Verification items for the finished model (mm, model axes). A direction names the side the tool comes from. Round coordinates to 2 decimals unless told otherwise and drop trailing zeros. Order: outer loops, then holes, each group sorted by start corner. A loop starts at its lowest first (then second) coordinate and runs counter-clockwise, first axis right, second up. Notation, with made-up numbers: M 74,13.25 L 117,13.25 A16 cw 117,43.25 Z; hole C 43,0 d1. An arc over 180 degrees is marked long. Use one line per item in the form item = value. Start each with the question number.
Item 1: Go/stop test with flat-tipped pins: pin 1 Ø0.5 at (y, z) = (4.5, 7.5) entering from +X; pin 2 Ø0.7 at (x, z) = (-4.5, 5) entering from +Y; pin 3 Ø2.5 at (x, z) = (0, 5) entering from +Y. Record where each tip stops, or that it passes through.
Item 2: Release check for a two-part mould opening along X. For faces 4 (the cylindrical face through (0.46, 2.47, 7.05)), 5 (the cylindrical face through (3.97, 1.97, 9.94)), 6 (the flat face through (1.3, 5, 2.8)) record: +X half, -X half, draft (parallel to the pull), parting line (faces both ways), or undercut.
Item 3: Thickness scan on probe 1 along Z at (x, y) = (0, 3.15); probe 2 along X at (y, z) = (2.05, 5); probe 3 along X at (y, z) = (3.75, 5). Record the ranges inside material, lowest first. Write a range as [from, to].
Item 4: Cross-section at B-B on z = 5. Enter the section's corners in (x, y), then the cut area to 3 significant figures.
Item 5: Tool access check on faces 1 (the flat face through (4, 4, 5)), 2 (the flat face through (0, 3, 10)), 3 (the flat face through (-4, 4, 5)). Record the directions out of +Z, -Z, +X, -X, +Y, -Y that give a thin tool (end or side, any length) a straight path to the whole face; none if there is none.
Item 6: Cross-section at C-C on z = 0.75. Enter the section's corners in (x, y), then the cut area to 3 significant figures.
Item 7: Cross-section at A-A on x = 0. Enter the section's corners in (y, z), then the cut area to 3 significant figures.
from build123d import *

# Parameters (mm, degrees)
NUTEXTRUSION_DEPTH    = 10
M5X0_8_TAPPED_HOLE1_D = 4.2
FILLET1_R             = 0.2


with BuildPart() as part:
    # MainSketch → NutExtrusion (new body)
    with BuildSketch(Plane.XY):
        Polygon((-3.1, 0), (3.1, 0), (5, 4), (3.1, 4), (3.1, 5), (-3.1, 5), (-3.1, 4), (-5, 4), align=None)
    extrude(amount=NUTEXTRUSION_DEPTH)

    # M5x0.8 Tapped Hole1 (through all)
    with Locations(Plane(origin=(0, 5, 0), x_dir=(1, 0, 0), z_dir=(0, 1, 0))):
        with Locations((0, -5)):
            Hole(M5X0_8_TAPPED_HOLE1_D / 2)

    # Fillet1
    fillet1_edges = [part.edges().sort_by_distance(p)[0] for p in [
        (4.05, 4, 0),
        (3.1, 4, 5),
        (3.1, 4.5, 0),
        (3.1, 5, 5),
        (0, 5, 0),
        (-3.1, 5, 5),
        (-3.1, 4.5, 0),
        (2.1, 5, 5),
        (2.1, 0, 5),
        (-3.1, 4, 5),
        (-4.05, 4, 0),
        (-5, 4, 5),
        (-4.05, 2, 0),
        (-3.1, 0, 5),
        (0, 0, 0),
        (0, 0, 10),
        (4.05, 2, 10),
        (4.05, 4, 10),
        (3.1, 4.5, 10),
        (0, 5, 10),
        (-3.1, 4.5, 10),
        (-4.05, 4, 10),
        (-4.05, 2, 10),
        (3.1, 0, 5),
        (4.05, 2, 0),
        (5, 4, 5),
    ]]
    fillet(fillet1_edges, radius=FILLET1_R)


solid = part.part
Output values:
q1.pin_1 = 3.1
q1.pin_2 = 4
q1.pin_3 = through
q2.face_4 = undercut
q2.face_5 = +X half
q2.face_6 = draft
q3.probe_1 = [0, 2.9], [7.1, 10]
q3.probe_2 = [-4.07, -2.1], [2.1, 4.07]
q3.probe_3 = [-4.88, -2.1], [2.1, 4.88]
q4.outline = M -4.86,3.71 L -3.15,0.11 A0.2 ccw -2.97,0 L -2.3,0 A0.2 ccw -2.1,0.2 L -2.1,4.8 A0.2 ccw -2.3,5 L -2.9,5 A0.2 ccw -3.1,4.8 L -3.1,4.2 A0.2 cw -3.3,4 L -4.68,4 A0.2 ccw Z; M 2.1,0.2 A0.2 ccw 2.3,0 L 2.97,0 A0.2 ccw 3.15,0.11 L 4.86,3.71 A0.2 ccw 4.68,4 L 3.3,4 A0.2 cw 3.1,4.2 L 3.1,4.8 A0.2 ccw 2.9,5 L 2.3,5 A0.2 ccw 2.1,4.8 Z
q4.area = 17.5 mm2
q5.face_1 = +Z, -Z, +X, +Y
q5.face_2 = +Z, +X, -X, +Y, -Y
q5.face_3 = +Z, -Z, -X, +Y
q6.outline = M -4.86,3.71 L -3.15,0.11 A0.2 ccw -2.97,0 L 2.97,0 A0.2 ccw 3.15,0.11 L 4.86,3.71 A0.2 ccw 4.68,4 L 3.3,4 A0.2 cw 3.1,4.2 L 3.1,4.8 A0.2 ccw 2.9,5 L -2.9,5 A0.2 ccw -3.1,4.8 L -3.1,4.2 A0.2 cw -3.3,4 L -4.68,4 A0.2 ccw Z
q6.area = 38.5 mm2
q7.outline = M 0,0.2 A0.2 ccw 0.2,0 L 4.8,0 A0.2 ccw 5,0.2 L 5,2.7 A0.2 ccw 4.8,2.9 L 0.2,2.9 A0.2 ccw 0,2.7 Z; M 0,7.3 A0.2 ccw 0.2,7.1 L 4.8,7.1 A0.2 ccw 5,7.3 L 5,9.8 A0.2 ccw 4.8,10 L 0.2,10 A0.2 ccw 0,9.8 Z
q7.area = 28.9 mm2
